The listing builds one solid part. Answer for the finished solid, in the listing's coordinates (mm). Face numbers are marked on the shaded views. A direction names the side the tool comes from. Round coordinates to 2 decimals unless told otherwise and drop trailing zeros. Loops run counter-clockwise (first coordinate to the right, second up) from the corner with the lowest first, then second, coordinate; pieces in that order, holes last. Notation, with made-up numbers: (44.25, 81) -> (68.25, 81) arc R12 cw to (68.25, 97) -> close; hole circle Ø4 at (-18, -31.5). An arc over 180 degrees is marked (long way). Use a Markdown table: item, result. Add a question column.
Q1. Section A-A on x = 0 is taken. Give the vertices of the cut face in (y, z).
Q2. Given pin 1 Ø5 at (x, y) = (5.5, -1) entering from -Z; pin 2 Ø2.5 at (x, z) = (0, 7) entering from -Y; pin 3 Ø2 at (x, z) = (3.5, -4) entering from +Y, each flat-ended and moving along its own axis, determine where each tip first touches the part or whether it passes through.
Q3. Section B-B on z = 0 is taken. Give the vertices of the cut face in (x, y), then the cut area to 3 significant figures.
Q4. Section D-D on z = -7 is taken. Give the vertices of the cut face in (x, y).
Q5. Consider line 1 (Z direction, x = 0, y = 0.8); line 2 (Y direction, x = -1.25, z = -3.75); line 3 (Y direction, x = 3.25, z = 0.25). Determine where each line is inside the solid, lowest interval first.
Q6. Section C-C on x = 7 is taken. Give the vertices of the cut face in (y, z).
Q7. Which of the six approach directions +Z, -Z, +X, -X, +Y, -Y give full straight-line access (tool end or side, diameter ignored) to the marked faces 5, 6 and 7?
Q8. For a pull along Z with two mould halves and no side action, classify the marked faces 1, 2, 3 and 4 as released by +Z, released by -Z, zero draft, split by the parting line, or undercut.
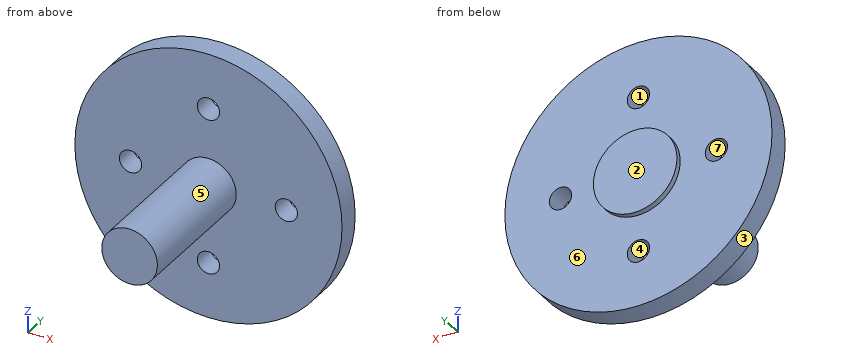
Autodesk Inventor part; units mm, degrees
ref_plane "YZ Plane" through (0, 0, 0) normal (1, 0, 0) x (0, 1, 0)
ref_plane "XZ Plane" through (0, 0, 0) normal (0, 1, 0) x (-1, 0, 0)
ref_plane "XY Plane" through (0, 0, 0) normal (0, 0, 1) x (1, 0, 0)
sketch "Sketch1" plane through (0, 0, 0) normal (0, 1, 0) x (-1, 0, 0)
  circle A0 centre (0, 0) radius 12
  dimension "sa_diameter" = 24
extrude "Extrusion1" add sketch "Sketch1" along normal blind 2
sketch "Sketch2" plane through (0, 0, 0) normal (0, -1, 0) x (1, 0, 0)
  circle A0 centre (0, 0) radius 2.5
  dimension "d4" = 5
extrude "Extrusion2" add sketch "Sketch2" along normal blind 12
sketch "Sketch4" plane through (0, 2, 0) normal (0, 1, 0) x (1, 0, 0)
  circle A0 centre (0, 0) radius 3.75
  dimension "d12" = 7.5
extrude "Extrusion4" add sketch "Sketch4" along normal blind 0.5
sketch "Sketch5" plane through (0, 2, 0) normal (0, 1, 0) x (1, 0, 0)
  circle A0 centre (0, 7) radius 1
  circle A1 centre (0, -7) radius 1
  circle A2 centre (-7, 0) radius 1
  circle A3 centre (7, 0) radius 1
  point P0 (0, 0)
  dimension "sa_hole_distance" = 7
  dimension "d16" = 7
  dimension "sa_hole_diameter" = 2
  dimension "d20" = 7
  dimension "d21" = 7
extrude "Extrusion5" cut sketch "Sketch5" against normal through all
equation "\"sa_diameter\" = servo_arm_diameter"
equation "\"sa_thickness\" = servo_arm_thickness"
equation "\"sa_hole_diameter\" = servo_arm_hole_diameter"
equation "\"servo_arm_thickness\" = 2"
equation "\"servo_arm_diameter\" = 24"
equation "\"servo_arm_hole_diameter\" = 2"
equation "\"servo_arm_hole_distance\" = 7"
properties part number "Servo_arm" material "ABS Plastic"
Checked values:
| question | item | result |
|---|---|---|
| 1 | outline | (-12, -2.5) -> (0, -2.5) -> (0, -6) -> (2, -6) -> (2, -3.75) -> (2.5, -3.75) -> (2.5, 3.75) -> (2, 3.75) -> (2, 6) -> (0, 6) -> (0, 2.5) -> (-12, 2.5) -> close; (0, -12) -> (2, -12) -> (2, -8) -> (0, -8) -> close; (0, 8) -> (2, 8) -> (2, 12) -> (0, 12) -> close |
| 2 | pin 1 | stops at z = -11.56 |
| 2 | pin 2 | stops at y = 0 |
| 2 | pin 3 | stops at y = 2 |
| 3 | outline | (-12, 0) -> (-8, 0) -> (-8, 2) -> (-12, 2) -> close; (-6, 0) -> (-2.5, 0) -> (-2.5, -12) -> (2.5, -12) -> (2.5, 0) -> (6, 0) -> (6, 2) -> (3.75, 2) -> (3.75, 2.5) -> (-3.75, 2.5) -> (-3.75, 2) -> (-6, 2) -> close; (8, 0) -> (12, 0) -> (12, 2) -> (8, 2) -> close |
| 3 | area | 104 mm2 |
| 4 | outline | (-9.75, 0) -> (-1, 0) -> (-1, 2) -> (-9.75, 2) -> close; (1, 0) -> (9.75, 0) -> (9.75, 2) -> (1, 2) -> close |
| 5 | line 1 | z = -12 to -8, -6 to 6, 8 to 12 |
| 5 | line 2 | y = 0 to 2 |
| 5 | line 3 | y = 0 to 2.5 |
| 6 | outline | (0, -9.75) -> (2, -9.75) -> (2, -1) -> (0, -1) -> close; (0, 1) -> (2, 1) -> (2, 9.75) -> (0, 9.75) -> close |
| 7 | face 5 | -Y |
| 7 | face 6 | +Y |
| 7 | face 7 | +Y, -Y |
| 8 | face 1 | undercut |
| 8 | face 2 | zero draft |
| 8 | face 3 | split by the parting line |
| 8 | face 4 | undercut |
